Design review of the part shown in the three views and the two pictorial views. Dimensions are in mm from the part's minimum x, y and z. Coordinates: 2 decimals unless noted, no trailing zeros. Write each loop counter-clockwise with the first axis right and the second up, starting at its lowest first coordinate (ties: lowest second). Pieces come first, ordered by that corner, then holes. Notation, with made-up numbers: M 13.25,-16 L 59.25,-16 A11 cw 59.25,-9 Z; hole C 30.5,41.25 d1. An arc over 180 degrees is marked long. One line per question, with ' | ' between items.
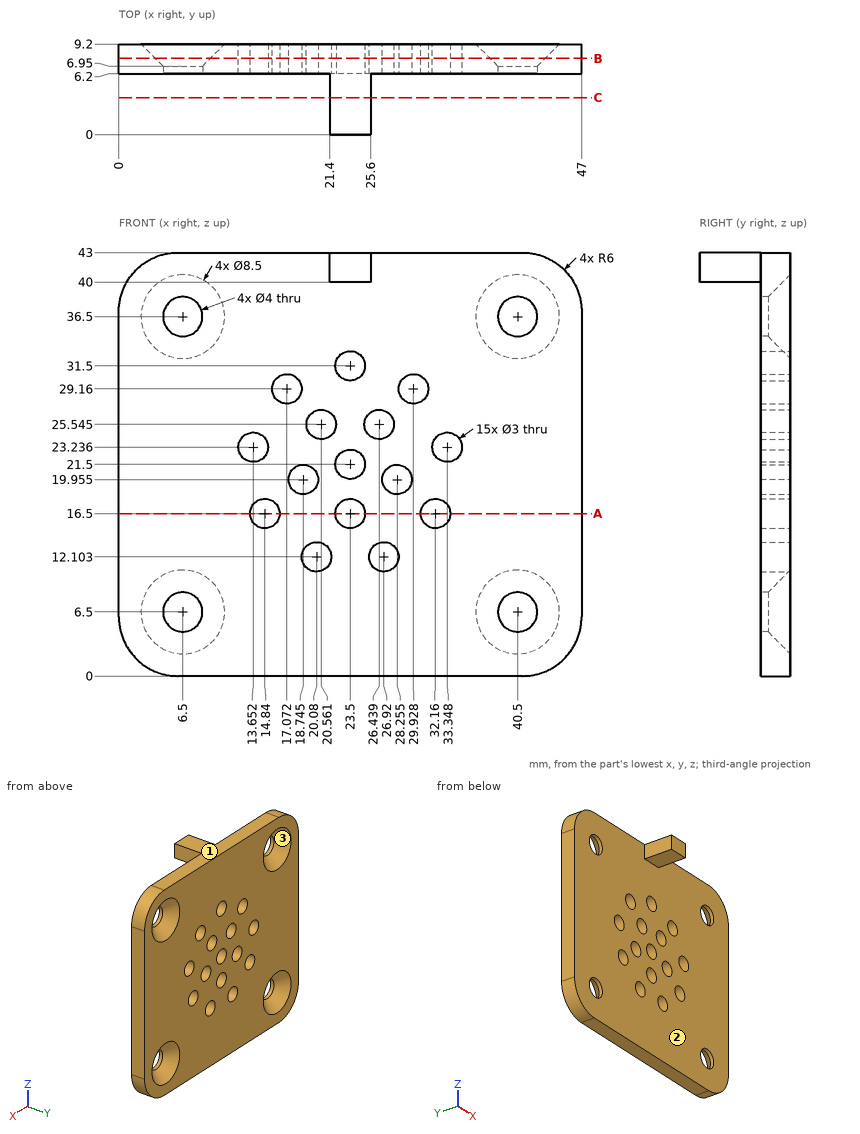
1. For line 1 along X through (y, z) = (6.6, 36.5); line 2 along Z through (x, y) = (40.5, 6.65); line 3 along X through (y, z) = (8.5, 29), list the stretches that pass through material, from the lowest coordinate up.
Computed values:
line 1: x = 0 to 4.5, 8.5 to 38.5, 42.5 to 47 | line 2: z = 0 to 4.5, 8.5 to 34.5, 38.5 to 43 | line 3: x = 0 to 15.58, 18.56 to 28.44, 31.42 to 47
2. Take a section at C-C on y = 3.75. State the section outline as (x, z) points, plus the area to 3 significant figures.
Computed values:
outline: M 21.4,40 L 25.6,40 L 25.6,43 L 21.4,43 Z | area: 12.6 mm2
3. Draft analysis for pull direction Z (two halves, no side actions). For the marked faces 1, 2 and 3, state which applies: pulls with the +Z half, pulls with the -Z half, needs draft (parallel to the pull), parting line crosses it, or undercut.
Computed values:
face 1: pulls with the +Z half | face 2: needs draft | face 3: undercut
4. Take a section at B-B on y = 7.75. Give the number of separate pieces and of enclosed holes in the cut face, plus the area to 3 significant figures.
Computed values:
separate pieces: 1 | enclosed holes: 19 | area: 1,790 mm2
5. Clearance check with flat-ended pins moving along their axes: P1, Ø21.5, axis at x = 33.5, z = 25, coming from the -Y side; P2, Ø3.5, axis at x = 23, y = 2.5, coming from the -Z side; P3, Ø2.5, axis at y = 3.5, z = 42, coming from the -X side; P4, Ø2.5, axis at x = 23.5, z = 16.5, coming from the -Y side. State where each tip first meets the part, or that it passes through.
Computed values:
P1: stops at y = 6.2 | P2: stops at z = 40 | P3: stops at x = 21.4 | P4: passes through
6. Take a section at A-A on z = 16.5. State the section outline as (x, y) points.
Computed values:
outline: M 0,6.2 L 13.34,6.2 L 13.34,9.2 L 0,9.2 Z; M 16.34,6.2 L 22,6.2 L 22,9.2 L 16.34,9.2 Z; M 25,6.2 L 30.66,6.2 L 30.66,9.2 L 25,9.2 Z; M 33.66,6.2 L 47,6.2 L 47,9.2 L 33.66,9.2 Z
